Drawing for the job (mm, zero at the part's lowest x, y, z). Round coordinates to 2 decimals unless told otherwise and drop trailing zeros. Write each loop counter-clockwise with the first axis right and the second up, starting at its lowest first coordinate (ties: lowest second). Pieces come first, ordered by that corner, then holes. Notation, with made-up numbers: M 10.5,-36 L 61.5,-36 A19 ccw 61.5,-23 Z; hole C 18,86 d4. An arc over 180 degrees is marked long. Use a Markdown table: item, result. Add a question column.
1) Slice it at C-C on x = 31.5. Write the cut outline in (y, z) (1 decimal), plus the area to 3 significant figures.
2) Slice it at D-D on y = 9. Write the cut outline in (x, z) (1 decimal).
3) Drop a flat-ended pin along its axis: P1, Ø4, axis at x = 64.5, y = 14, coming from the -Z side. Give the stop position or say it passes through.
4) Slice it at B-B on z = 2.9. Write the cut outline in (x, y) (1 decimal), plus the area to 3 significant figures.
5) Wall check: probe 1 along Y at (x, z) = (43, 1.1); probe 2 along X at (y, z) = (11, 2.2) (1 decimal); probe 3 along X at (y, z) = (17.5, 1.75). Give the ranges that are in metal, low to high.
6) Slice it at A-A on y = 4. Write the cut outline in (x, z) (1 decimal).
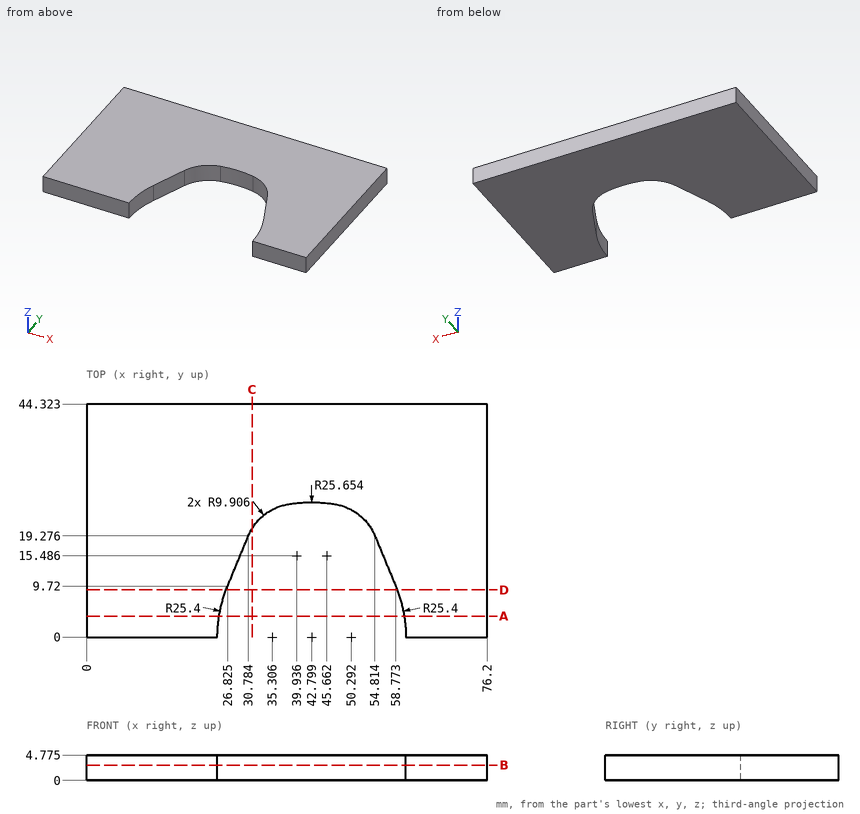
Entries:
| question | item | result |
|---|---|---|
| 1 | outline | M 20.7,0 L 44.3,0 L 44.3,4.8 L 20.7,4.8 Z |
| 1 | area | 113 mm^2 |
| 2 | outline | M 0,0 L 26.5,0 L 26.5,4.8 L 0,4.8 Z; M 59.1,0 L 76.2,0 L 76.2,4.8 L 59.1,4.8 Z |
| 3 | P1 | stops at z = 0 |
| 4 | outline | M 0,0 L 24.9,0 A25.4 cw 26.8,9.7 L 30.8,19.3 A9.9 cw 38.1,25.2 A25.7 cw 47.5,25.2 A9.9 cw 54.8,19.3 L 58.8,9.7 A25.4 cw 60.7,0 L 76.2,0 L 76.2,44.3 L 0,44.3 Z |
| 4 | area | 2,660 mm^2 |
| 5 | probe 1 | y = 25.65 to 44.32 |
| 5 | probe 2 | x = 0 to 27.4, 58.2 to 76.2 |
| 5 | probe 3 | x = 0 to 30.05, 55.55 to 76.2 |
| 6 | outline | M 0,0 L 25.2,0 L 25.2,4.8 L 0,4.8 Z; M 60.4,0 L 76.2,0 L 76.2,4.8 L 60.4,4.8 Z |
